```python
from build123d import *

# Parameters (mm, degrees)
SKIZZE1_W                       = 500
SKIZZE1_H                       = 360
AUFSATZ_LINEAR_AUSTRAGEN1_DEPTH = 20
FASE1_SIZE                      = 10
SKIZZE3_R                       = 2
SCHNITT_LINEAR_AUSTRAGEN1_DEPTH = 309.706980809


with BuildPart() as part:
    # Skizze1 → Aufsatz-Linear austragen1 (new body)
    with BuildSketch(Plane(origin=(0, 0, 0), x_dir=(1, 0, 0), z_dir=(0, 1, 0))):
        Rectangle(SKIZZE1_W, SKIZZE1_H)
    extrude(amount=AUFSATZ_LINEAR_AUSTRAGEN1_DEPTH)

    # Fase1
    fase1_edges = [part.edges().sort_by_distance(p)[0] for p in [
        (0, 20, 180),
        (-250, 20, 0),
        (0, 20, -180),
        (250, 20, 0),
        (0, 0, -180),
        (-250, 0, 0),
        (0, 0, 180),
        (250, 0, 0),
    ]]
    chamfer(fase1_edges, length=FASE1_SIZE - 0.0001)  # a hair under: the kernel refuses the full size

    # Skizze3 → Schnitt-Linear austragen1 (cut, through all)
    with BuildSketch(Plane(origin=(0, 20, 0), x_dir=(1, 0, 0), z_dir=(0, 1, 0))):
        with Locations(Location((-227.5, 157.5, 0), (0, 0, 270))):
            Circle(SKIZZE3_R)
        with Locations(Location((-102.5, 157.5, 0), (0, 0, 270))):
            Circle(SKIZZE3_R)
        with Locations(Location((142.5, 157.5, 0), (0, 0, 270))):
            Circle(SKIZZE3_R)
        with Locations(Location((227.5, 157.5, 0), (0, 0, 270))):
            Circle(SKIZZE3_R)
        with Locations(Location((227.5, -157.5, 0), (0, 0, 270))):
            Circle(SKIZZE3_R)
        with Locations(Location((142.5, -157.5, 0), (0, 0, 270))):
            Circle(SKIZZE3_R)
        with Locations(Location((-102.5, -157.5, 0), (0, 0, 270))):
            Circle(SKIZZE3_R)
        with Locations(Location((-227.5, -157.5, 0), (0, 0, 270))):
            Circle(SKIZZE3_R)
    extrude(amount=-SCHNITT_LINEAR_AUSTRAGEN1_DEPTH, mode=Mode.SUBTRACT)


solid = part.part
```
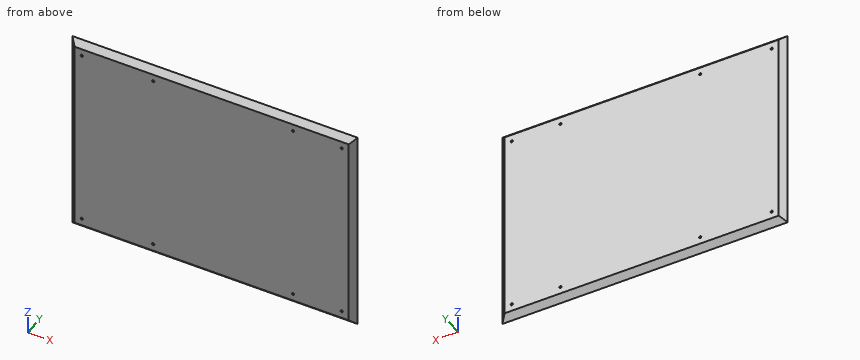
Can you work these out from the model? Positions are in its coordinate system, mm. Round coordinates to 2 decimals unless told otherwise and drop trailing zeros. Return JSON: item names as keys, results as strings. Group by question number.
1. Will these pins go through, and if not, where does the flat tip stop? pin 1 (3.5 mm diameter, centred on x = -227.5, z = 157.5, fed in from -Y); pin 2 (1 mm diameter, centred on y = 9, z = -120, fed in from -X); pin 3 (2 mm diameter, centred on y = 11.5, z = 123, fed in from +X); pin 4 (1.5 mm diameter, centred on x = -73.5, y = 15.5, fed in from -Z).
2. I need wall thicknesses on line 1 (X direction, y = 13.75, z = 157.5); line 2 (X direction, y = 13, z = 157.5); line 3 (Z direction, x = 142.5, y = 16.25). Which ranges of each line are inside material? Lowest first, please. Write a range as [from, to].
3. If we section it at A-A, the plane y = 6.75: Count the separate pieces of the cut face and the enclosed holes in it, then the cut area to 3 significant figures.
Output values:
{
 "1": {"pin 1": "through", "pin 2": "x = -249.5", "pin 3": "x = 249.5", "pin 4": "z = -175.25"},
 "2": {"line 1": "[-246.25, -229.5], [-225.5, -104.5], [-100.5, 140.5], [144.5, 225.5], [229.5, 246.25]", "line 2": "[-247, -229.5], [-225.5, -104.5], [-100.5, 140.5], [144.5, 225.5], [229.5, 247]", "line 3": "[-173.75, -159.5], [-155.5, 155.5], [159.5, 173.75]"},
 "3": {"separate pieces": "1", "enclosed holes": "8", "area": "174,000 mm²"}
}
